The drawing under review shows one solid part. Ordinate dimensions are in mm from its lowest x, y, z. A direction names the side the tool comes from. Round coordinates to 2 decimals unless told otherwise and drop trailing zeros. Loops run counter-clockwise (first coordinate to the right, second up) from the corner with the lowest first, then second, coordinate; pieces in that order, holes last. Notation, with made-up numbers: (1, -18.75) - (35, -18.75) arc R33 cw to (35, 20.25) - close; hole circle Ø10 at (-7.75, -11.5). An arc over 180 degrees is marked (long way). Answer as CSV lines item,"result".
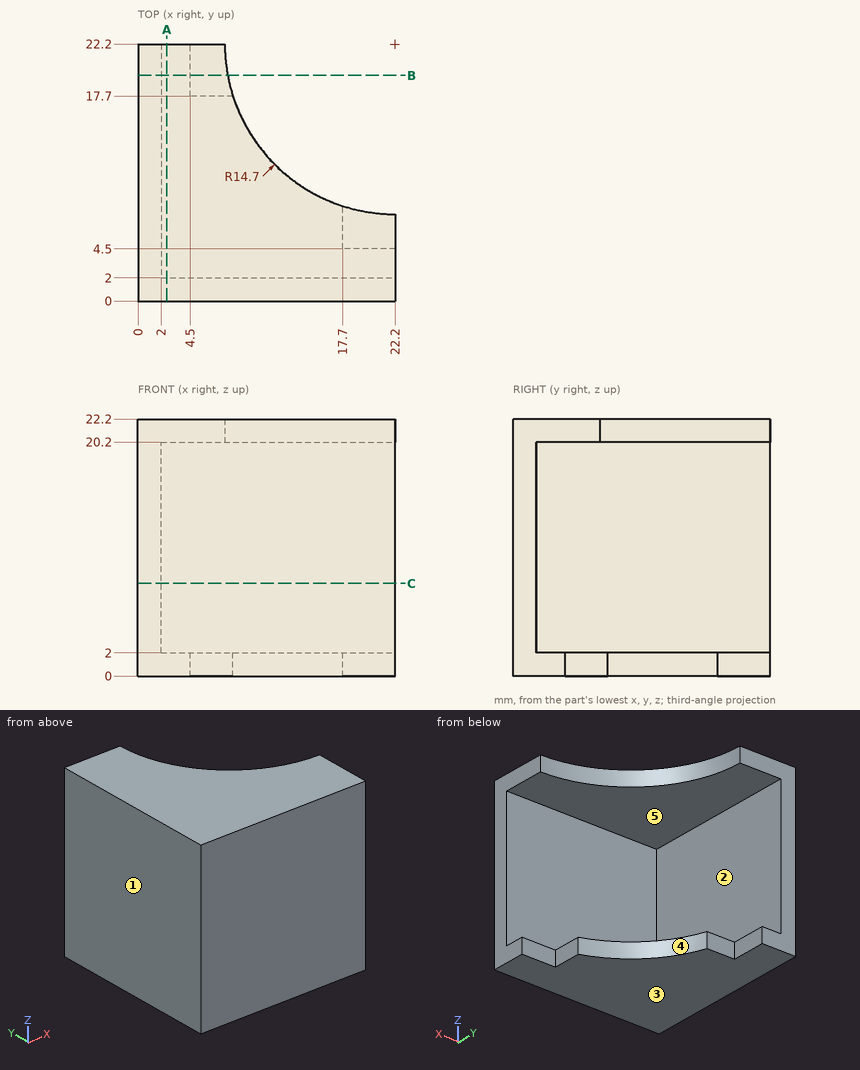
1. Tool access review of the marked faces 4 and 5: name each direction out of +Z, -Z, +X, -X, +Y, -Y from which nothing blocks a thin tool from reaching the whole face with its end or side.
Numbers:
face 4,"+Z, -Z, +X, +Y"
face 5,"+X, +Y"
2. Clearance check with flat-ended pins moving along their axes: pin 1 (8 mm diameter, centred on x = 7, y = 10.5, fed in from -Z); pin 2 (5 mm diameter, centred on y = 11.5, z = 13, fed in from +X); pin 3 (1.6 mm diameter, centred on x = 20, z = 0.5, fed in from +Y); pin 4 (0.6 mm diameter, centred on y = 19.5, z = 0.5, fed in from +X). State where each tip first meets the part, or that it passes through.
Numbers:
pin 1,"stops at z = 0"
pin 2,"stops at x = 2"
pin 3,"stops at y = 4.5"
pin 4,"stops at x = 4.5"
3. Take a section at B-B (y = 19.5). State the section outline as (x, z) points, plus the area to 3 significant figures.
Numbers:
outline,"(0, 0) - (4.5, 0) - (4.5, 2) - (2, 2) - (2, 20.2) - (7.75, 20.2) - (7.75, 22.2) - (0, 22.2) - close"
area,"60.9 mm²"
4. Take a section at A-A (x = 2.5). State the section outline as (y, z) points, plus the area to 3 significant figures.
Numbers:
outline,"(0, 0) - (22.2, 0) - (22.2, 2) - (2, 2) - (2, 20.2) - (22.2, 20.2) - (22.2, 22.2) - (0, 22.2) - close"
area,"125 mm²"
5. Draft analysis for pull direction Z (two halves, no side actions). For the marked faces 1, 2 and 3, state which applies: +Z half, -Z half, draft (parallel to the pull), parting line (faces both ways), or undercut.
Numbers:
face 1,"draft"
face 2,"undercut"
face 3,"-Z half"
6. Take a section at C-C (z = 8). State the section outline as (x, y) points, plus the area to 3 significant figures.
Numbers:
outline,"(0, 0) - (22.2, 0) - (22.2, 2) - (2, 2) - (2, 22.2) - (0, 22.2) - close"
area,"84.8 mm²"
7. Wall thickness on probe 1 along Z at (x, y) = (4, 11.5); probe 2 along X at (y, z) = (4.5, 11.25): over which ranges is each line inside the solid? List them lowest first.
Numbers:
probe 1,"z = 0 to 2, 20.2 to 22.2"
probe 2,"x = 0 to 2"
